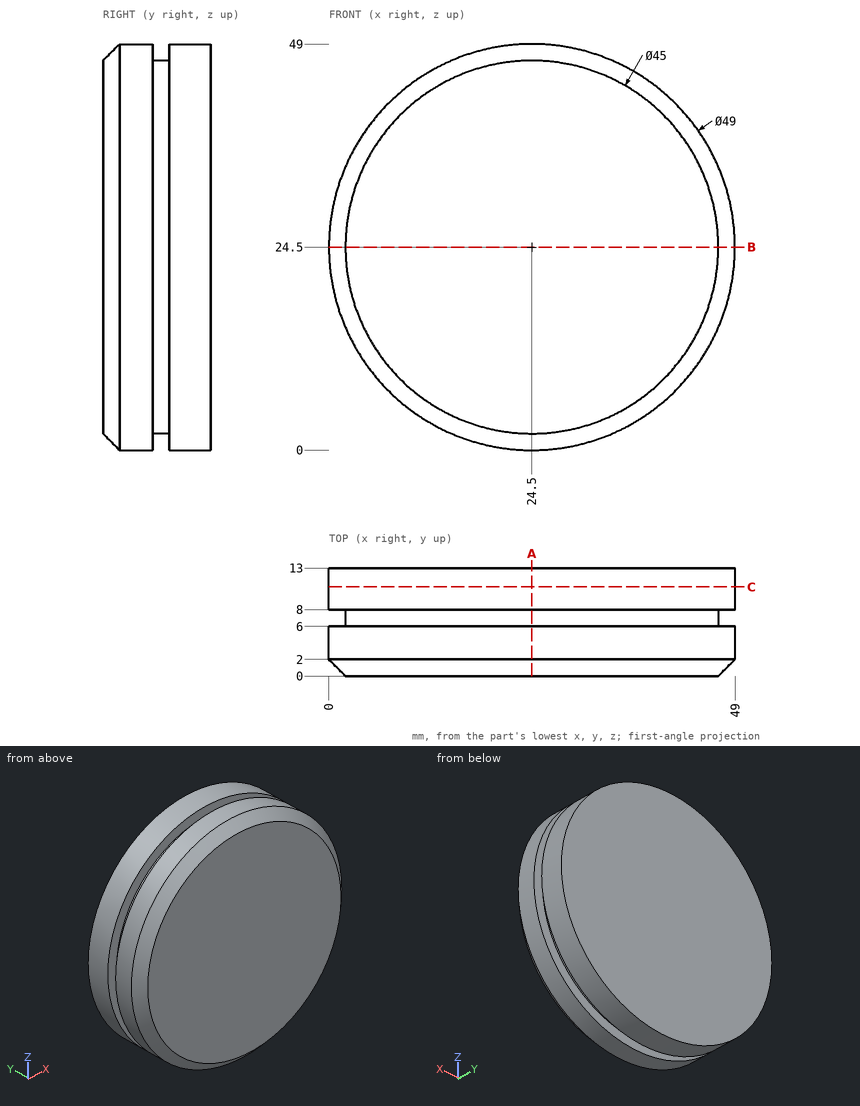
Print and shaded views of the part. All mm, measured from the part's lowest x, y and z. Round coordinates to 2 decimals unless told otherwise and drop trailing zeros. Write each loop counter-clockwise with the first axis right and the second up, starting at its lowest first coordinate (ties: lowest second). Pieces come first, ordered by that corner, then holes. Notation, with made-up numbers: (-21.5, 31.25) -> (-4.5, 31.25) arc R23 cw to (-4.5, 69.25) -> close; hole circle Ø3 at (15, 56.25). An arc over 180 degrees is marked (long way). Write item = value, one per line.
(1) Band-saw the part on B-B (z = 24.5). Give the cut face in (x, y), then the cut area to 3 significant figures.
Answer:
outline = (0, 2) -> (2, 0) -> (47, 0) -> (49, 2) -> (49, 6) -> (47, 6) -> (47, 8) -> (49, 8) -> (49, 13) -> (0, 13) -> (0, 8) -> (2, 8) -> (2, 6) -> (0, 6) -> close
area = 625 mm2
(2) Probe L1, parallel to X at y = 1.75, z = 6.5; L2, parallel to X at y = 3.25, z = 44; L3, parallel to Z at x = 18, y = 7.5. List the from-to ranges inside material, lowest first.
Answer:
L1 = 8.25 to 40.75
L2 = 9.67 to 39.33
L3 = 2.96 to 46.04
(3) Band-saw the part on A-A (x = 24.5). Give the cut face in (y, z).
Answer:
outline = (0, 2) -> (2, 0) -> (6, 0) -> (6, 2) -> (8, 2) -> (8, 0) -> (13, 0) -> (13, 49) -> (8, 49) -> (8, 47) -> (6, 47) -> (6, 49) -> (2, 49) -> (0, 47) -> close
(4) Flat gauge pins, fed straight in: pin 1 (4 mm diameter, centred on x = 35.5, y = 4, fed in from +Z); pin 2 (5 mm diameter, centred on y = 2.5, z = 42.5, fed in from -X); pin 3 (4 mm diameter, centred on x = 36.5, y = 2, fed in from +Z). Where does each tip first touch, or does it go through?
Answer:
pin_1 = 47.29
pin_2 = 5.53
pin_3 = 46.87
(5) Band-saw the part on C-C (y = 10.75). Give the cut face in (x, z), then the cut area to 3 significant figures.
Answer:
outline = circle Ø49 at (24.5, 24.5)
area = 1,890 mm2
